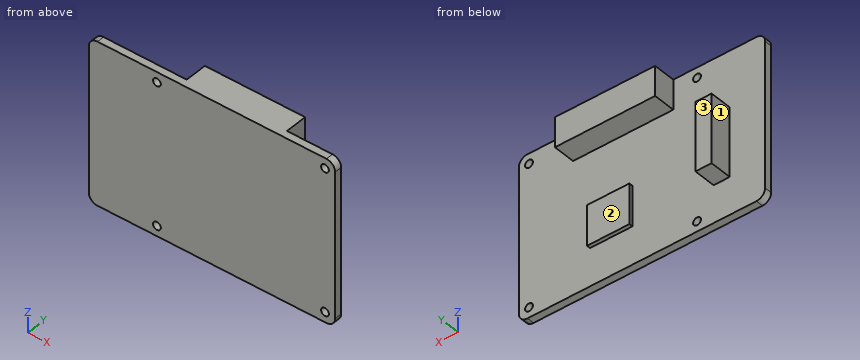
from build123d import *

# Parameters (mm, degrees)
SKETCH1_R           = 2.999997759
SKETCH1_R_2         = 1.35
BOSS_EXTRUDE1_DEPTH = 2.54
SKETCH2_W           = 34.5908584
SKETCH2_H           = 10.2596717
BOSS_EXTRUDE2_DEPTH = 7.62
SKETCH3_W           = 5.570985132
SKETCH3_H           = 23.769243549
BOSS_EXTRUDE3_DEPTH = 7.62
SKETCH4_W           = 14.639482868
SKETCH4_H           = 13.879415804
BOSS_EXTRUDE4_DEPTH = 1.27


with BuildPart() as part:
    # Sketch1 → Boss-Extrude1 (new body)
    # profile 1 of 5: a face of its own
    with BuildSketch(Plane(origin=(0, 0, 0), x_dir=(1, 0, 0), z_dir=(0, 1, 0))):
        with BuildLine():
            Line((-39.500002241, -28), (39.500002241, -28))
            ThreePointArc((39.500002241, -28), (41.621321, -27.121321), (42.5, -25.000002241))
            Line((42.5, -25.000002241), (42.5, 25.000002241))
            ThreePointArc((42.5, 25.000002241), (41.621321, 27.121321), (39.500002241, 28))
            Line((39.500002241, 28), (-39.500002241, 28))
            ThreePointArc((-39.500002241, 28), (-41.621321, 27.121321), (-42.5, 25.000002241))
            Line((-42.5, 25.000002241), (-42.5, -25.000002241))
            ThreePointArc((-42.5, -25.000002241), (-41.621321, -27.121321), (-39.500002241, -28))
        make_face()
        with Locations((39, 24.5)):
            Circle(SKETCH1_R, mode=Mode.SUBTRACT)
        with Locations((-19, -24.5)):
            Circle(SKETCH1_R, mode=Mode.SUBTRACT)
        with Locations((-19, 24.5)):
            Circle(SKETCH1_R, mode=Mode.SUBTRACT)
        with Locations((39, -24.5)):
            Circle(SKETCH1_R, mode=Mode.SUBTRACT)
    # profile 2 of 5: a face of its own
    with BuildSketch(Plane(origin=(0, 0, 0), x_dir=(1, 0, 0), z_dir=(0, 1, 0))):
        with Locations((-19, 24.5)):
            Circle(SKETCH1_R)
        with Locations(Location((-19, 24.5, 0), (0, 0, 270))):
            Circle(SKETCH1_R_2, mode=Mode.SUBTRACT)
    # profile 3 of 5: a face of its own
    with BuildSketch(Plane(origin=(0, 0, 0), x_dir=(1, 0, 0), z_dir=(0, 1, 0))):
        with Locations((-19, -24.5)):
            Circle(SKETCH1_R)
        with Locations(Location((-19, -24.5, 0), (0, 0, 270))):
            Circle(SKETCH1_R_2, mode=Mode.SUBTRACT)
    # profile 4 of 5: a face of its own
    with BuildSketch(Plane(origin=(0, 0, 0), x_dir=(1, 0, 0), z_dir=(0, 1, 0))):
        with Locations((39, 24.5)):
            Circle(SKETCH1_R)
        with Locations(Location((39, 24.5, 0), (0, 0, 270))):
            Circle(SKETCH1_R_2, mode=Mode.SUBTRACT)
    # profile 5 of 5: a face of its own
    with BuildSketch(Plane(origin=(0, 0, 0), x_dir=(1, 0, 0), z_dir=(0, 1, 0))):
        with Locations((39, -24.5)):
            Circle(SKETCH1_R)
        with Locations(Location((39, -24.5, 0), (0, 0, 270))):
            Circle(SKETCH1_R_2, mode=Mode.SUBTRACT)
    extrude(amount=BOSS_EXTRUDE1_DEPTH)

    # Sketch2 → Boss-Extrude2 (add)
    with BuildSketch(Plane(origin=(0, 2.54, 0), x_dir=(1, 0, 0), z_dir=(0, 1, 0))):
        with Locations((6.499175034, -22.87016415)):
            Rectangle(SKETCH2_W, SKETCH2_H)
    extrude(amount=BOSS_EXTRUDE2_DEPTH)

    # Sketch3 → Boss-Extrude3 (add)
    with BuildSketch(Plane(origin=(0, 2.54, 0), x_dir=(1, 0, 0), z_dir=(0, 1, 0))):
        with Locations((-27.506444174, 3.193413678)):
            Rectangle(SKETCH3_W, SKETCH3_H)
    extrude(amount=BOSS_EXTRUDE3_DEPTH)

    # Sketch4 → Boss-Extrude4 (add)
    with BuildSketch(Plane(origin=(0, 2.54, 0), x_dir=(1, 0, 0), z_dir=(0, 1, 0))):
        with Locations((10.616389604, 7.997233107)):
            Rectangle(SKETCH4_W, SKETCH4_H)
    extrude(amount=BOSS_EXTRUDE4_DEPTH)


solid = part.part
Input: part model. Units: mm. Frame: model coordinates. Face numbers are marked on the shaded views. A direction names the side the tool comes from. Give positions to 0.01 mm unless a question says otherwise; leave off trailing zeros. Write each loop counter-clockwise with the first axis right and the second up, starting at its lowest first coordinate (ties: lowest second). Pieces come first, ordered by that corner, then holes.
Q1. Section C-C, the plane z = -10. Output: boundary loops of the cut face in (x, y), plus the area to 3 significant figures.
Q2. Set-up query: the marked faces 1, 2 and 3. Return all of +Z, -Z, +X, -X, +Y, -Y with unobstructed straight access to the full face (end or side cutting, diameter ignored); none if empty.
Q3. Material intervals for probe 1 along X at (y, z) = (1.85, 24.5); probe 2 along Y at (x, z) = (15.5, -12.5); probe 3 along X at (y, z) = (4.75, -9), sorted ascending.
Q4. First-contact query: P1, Ø0.6, axis at x = 7, y = 3, coming from the -Z side; P2, Ø4.5, axis at x = 39, z = -24.5, coming from the +Y side; P3, Ø6, axis at x = -28.5, y = 7.5, coming from the -Z side. Flat tips, straight axial feed; report the tip coordinate or a pass-through.
Q5. Section A-A, the plane y = 8.5. Output: boundary loops of the cut face in (x, z).
Q6. Section B-B, the plane x = -19. Output: boundary loops of the cut face in (y, z).
Q7. Section D-D, the plane x = 13. Output: boundary loops of the cut face in (y, z).
Filled in:
1. outline: (-42.5, 0) - (42.5, 0) - (42.5, 2.54) - (17.94, 2.54) - (17.94, 3.81) - (3.3, 3.81) - (3.3, 2.54) - (-24.72, 2.54) - (-24.72, 10.16) - (-30.29, 10.16) - (-30.29, 2.54) - (-42.5, 2.54) - close
1. area: 277 mm2
2. face 1: +Z, -Z, -X, +Y
2. face 2: -Z, +X, +Y
2. face 3: +Z, -Z, +X, -X, +Y
3. probe 1: x = -42.5 to -20.35, -17.65 to 37.65, 40.35 to 42.5
3. probe 2: y = 0 to 3.81
3. probe 3: x = -30.29 to -24.72
4. P1: stops at z = -14.94
4. P2: stops at y = 2.54
4. P3: stops at z = -15.08
5. outline: (-30.29, -15.08) - (-24.72, -15.08) - (-24.72, 8.69) - (-30.29, 8.69) - close; (-10.8, 17.74) - (23.79, 17.74) - (23.79, 28) - (-10.8, 28) - close
6. outline: (0, -28) - (2.54, -28) - (2.54, -25.85) - (0, -25.85) - close; (0, -23.15) - (2.54, -23.15) - (2.54, 23.15) - (0, 23.15) - close; (0, 25.85) - (2.54, 25.85) - (2.54, 28) - (0, 28) - close
7. outline: (0, -28) - (2.54, -28) - (2.54, -14.94) - (3.81, -14.94) - (3.81, -1.06) - (2.54, -1.06) - (2.54, 17.74) - (10.16, 17.74) - (10.16, 28) - (0, 28) - close
